Autodesk Fusion 360 part; units mm, degrees
sketch "Sketch1" plane through (0, 0, 0) normal (0, 0, 1) x (1, 0, 0)
  line L0 (0, 0) -> (80, 0)
  line L1 (80, 0) -> (80, 80)
  line L2 (80, 80) -> (0, 80)
  line L3 (0, 80) -> (0, 0)
  line L4 (0, 20) -> (20, 0)
  circle A0 centre (40, 40) radius 15
  dimension "d1" = 80
  dimension "d2" = 80
  dimension "d3" = 20
  dimension "d4" = 20
  dimension "d5" = 30
  dimension "d6" = 40
  dimension "d7" = 40
extrude "Extrude1" add sketch "Sketch1" along normal blind 10 contours L0 L1 L2 L3 L4
sketch "Sketch2" plane through (0, 0, 10) normal (0, 0, 1) x (-1, 0, 0)
  circle A0 centre (-40, -40) radius 15
  line L0 (0, -20) -> (-20, 0)
  line L1 (-20, 0) -> (-80, 0)
  line L2 (-80, 0) -> (-80, -80)
  line L3 (-80, -80) -> (0, -80)
  line L4 (0, -80) -> (0, -20)
  line L5 (0, -80) -> (-80, -80)
  line L6 (-80, -80) -> (-80, -70)
  line L7 (-80, -70) -> (0, -70)
  line L8 (0, -70) -> (0, -80)
  line L9 (-80, 0) -> (-70, 0)
  line L10 (-70, 0) -> (-70, -80)
  line L11 (-70, -80) -> (-80, -80)
  line L12 (-80, -80) -> (-80, 0)
  dimension "d10" = 10
  dimension "d11" = 10
extrude "Extrude2" add sketch "Sketch2" along normal blind 40 contours L3 L4 L5 L7 L8 L10 | L1 L2 L7 L9 L10 L12 | L2 L3 L5 L6 L7 L10 L11 L12
fillet "Fillet1" radius 4 1 edges at (80, 80, 25)
sketch "Sketch3" plane through (80, 0, 0) normal (1, 0, 0) x (0, 1, 0)
  line L0 (76, 0) -> (76, 50)
  line L1 (76, 50) -> (0, 50)
  line L2 (0, 50) -> (0, 0)
  line L3 (0, 0) -> (76, 0)
  circle A0 centre (35, 30) radius 7.5
  line L4 (0, 10) -> (70, 10)
  dimension "d16" = 15
  dimension "d17" = 35
  dimension "d18" = 20
extrude "Extrude3" cut sketch "Sketch3" against normal blind 10 contours A0
sketch "Sketch5" plane through (0, 70, 0) normal (0, -1, 0) x (1, 0, 0)
  line L0 (0, 10) -> (70, 10)
  line L1 (70, 10) -> (70, 50)
  line L2 (70, 50) -> (0, 50)
  line L3 (0, 50) -> (0, 10)
  circle A0 centre (35, 30) radius 7.5
  dimension "d24" = 15
  dimension "d25" = 35
  dimension "d26" = 20
extrude "Extrude4" cut sketch "Sketch5" against normal blind 10 contours A0
sketch "Sketch6" plane through (0, 0, 10) normal (0, 0, 1) x (-1, 0, 0)
  line L0 (-70, -70) -> (0, -70)
  line L1 (0, -70) -> (0, -20)
  line L2 (0, -20) -> (-20, 0)
  line L3 (-20, 0) -> (-70, 0)
  line L4 (-70, 0) -> (-70, -70)
  circle A0 centre (-40, -40) radius 15
sketch "Sketch4" plane through (0, 70, 0) normal (0, -1, 0) x (1, 0, 0)
  line L0 (0, 10) -> (70, 10)
  line L1 (70, 10) -> (70, 50)
  line L2 (70, 50) -> (0, 50)
  line L3 (0, 50) -> (0, 10)
  circle A0 centre (35, 30) radius 7.5
  dimension "d21" = 15
  dimension "d22" = 35
  dimension "d23" = 20
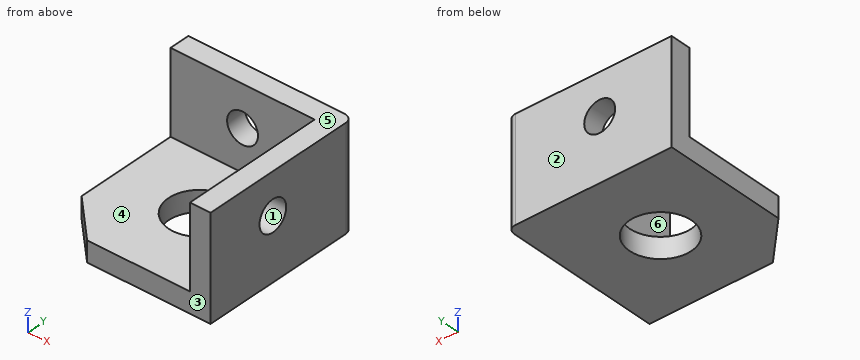
Read the model definition and answer for the solid it produces. Units are mm, in the model's axes. Face numbers are marked on the shaded views. A direction names the side the tool comes from. Give positions to 0.01 mm unless a question says otherwise; leave off trailing zeros. Write each loop counter-clockwise with the first axis right and the second up, starting at its lowest first coordinate (ties: lowest second). Pieces come first, ordered by that corner, then holes. Notation, with made-up numbers: (76.5, 2.5) - (97.5, 2.5) arc R21 ccw to (97.5, 37.5) - close; hole circle Ø1 at (-14.75, -14.5). An arc over 180 degrees is marked (long way). Use CSV: the item, a comma, the result in double quotes. Start each with the question number.
(1) Given P1, Ø1, axis at y = 46.5, z = 13, coming from the -X side; P2, Ø2, axis at x = 9.5, z = 16.5, coming from the -Y side; P3, Ø4, axis at x = 21.5, y = 19, coming from the +Z side, each flat-ended and moving along its own axis, determine where each tip first touches the part or whether it passes through.
(2) Find section A-A (z = 5). Give the vertices of the cut face in (x, y).
(3) For the marked faces 5 and 6, determine the directions among +Z, -Z, +X, -X, +Y, -Y from which every point of the face is accessible in a straight line to the end or side of a thin tool.
(4) Determine the mould class of the marked faces 1, 2, 3 and 4 for opening direction Y: +Y half, -Y half, draft (parallel to the pull), parting line (faces both ways), or undercut.
(5) Find section C-C (z = 30). Give the vertices of the cut face in (x, y), plus the area to 3 significant figures.
(6) Consider line 1 along Z through (x, y) = (77.75, 35); line 2 along X through (y, z) = (57, 41.5); line 3 along Z through (x, y) = (12.5, 61). Determine where each line is inside the solid, lowest interval first.
(7) Find section B-B (x = 35). Give the vertices of the cut face in (y, z).
Findings below:
1,P1,"x = 70"
1,P2,"y = 70"
1,P3,"z = 10"
2,outline,"(0, 20) - (20, 0) - (80, 0) - (80, 76) arc R4 ccw to (76, 80) - (0, 80) - close; hole circle Ø30 at (40, 40)"
3,face 5,"+Z, +X, -X, +Y, -Y"
3,face 6,"+Z, -X, -Y"
4,face 1,"undercut"
4,face 2,"+Y half"
4,face 3,"-Y half"
4,face 4,"draft"
5,outline,"(0, 70) - (27.5, 70) - (27.5, 80) - (0, 80) - close; (42.5, 70) - (70, 70) - (70, 42.5) - (80, 42.5) - (80, 76) arc R4 ccw to (76, 80) - (42.5, 80) - close; (70, 0) - (80, 0) - (80, 27.5) - (70, 27.5) - close"
5,area,"1,200 mm2"
6,line 1,"0 to 22.5, 37.5 to 50"
6,line 2,"70 to 80"
6,line 3,"0 to 10"
7,outline,"(0, 0) - (25.86, 0) - (25.86, 10) - (0, 10) - close; (54.14, 0) - (80, 0) - (80, 22.5) - (70, 22.5) - (70, 10) - (54.14, 10) - close; (70, 37.5) - (80, 37.5) - (80, 50) - (70, 50) - close"
